from build123d import *

# Parameters (mm, degrees)
SKIZZE1_W                       = 35
SKIZZE1_H                       = 35
AUFSATZ_LINEAR_AUSTRAGEN1_DEPTH = 34
SKIZZE2_R                       = 16
AUFSATZ_LINEAR_AUSTRAGEN2_DEPTH = 35.8
SKIZZE3_R                       = 9.5
AUFSATZ_LINEAR_AUSTRAGEN3_DEPTH = 2
SKIZZE4_R                       = 3
AUFSATZ_LINEAR_AUSTRAGEN4_DEPTH = 18
SKIZZE5_R                       = 1.5
SCHNITT_LINEAR_AUSTRAGEN1_DEPTH = 4
FASE1_SIZE                      = 3
AUFSATZ_LINEAR_START            = 0.5
AUFSATZ_LINEAR_AUSTRAGEN5_DEPTH = 4.5
SCHNITT_LINEAR_AUSTRAGEN2_DEPTH = 12


with BuildPart() as part:
    # Skizze1 → Aufsatz-Linear austragen1 (new body)
    with BuildSketch(Plane.XY):
        Rectangle(SKIZZE1_W, SKIZZE1_H)
    extrude(amount=AUFSATZ_LINEAR_AUSTRAGEN1_DEPTH)

    # Skizze2 → Aufsatz-Linear austragen2 (add)
    with BuildSketch(Plane.XY.offset(34)):
        Circle(SKIZZE2_R)
    extrude(amount=AUFSATZ_LINEAR_AUSTRAGEN2_DEPTH)

    # Skizze3 → Aufsatz-Linear austragen3 (add)
    with BuildSketch(Plane.XY.offset(69.8)):
        Circle(SKIZZE3_R)
    extrude(amount=AUFSATZ_LINEAR_AUSTRAGEN3_DEPTH)

    # Skizze4 → Aufsatz-Linear austragen4 (add)
    with BuildSketch(Plane.XY.offset(69.8)):
        Circle(SKIZZE4_R)
    extrude(amount=AUFSATZ_LINEAR_AUSTRAGEN4_DEPTH)

    # Skizze5 → Schnitt-Linear austragen1 (cut)
    with BuildSketch(Plane.XY.offset(69.8)):
        with Locations((0, 13)):
            Circle(SKIZZE5_R)
        with Locations((13, 0)):
            Circle(SKIZZE5_R)
        with Locations((-13, 0)):
            Circle(SKIZZE5_R)
        with Locations((0, -13)):
            Circle(SKIZZE5_R)
    extrude(amount=-SCHNITT_LINEAR_AUSTRAGEN1_DEPTH, mode=Mode.SUBTRACT)

    # Fase1
    fase1_edges = [part.edges().sort_by_distance(p)[0] for p in [
        (-17.5, 17.5, 17),
        (17.5, 17.5, 17),
        (17.5, -17.5, 17),
        (-17.5, -17.5, 17),
    ]]
    chamfer(fase1_edges, length=FASE1_SIZE)

    # Skizze6 → Aufsatz-Linear austragen5 (add)
    with BuildSketch(Plane.XY.offset(34).offset(AUFSATZ_LINEAR_START)):
        Polygon((-17.5, 14.5), (-17.5, -14.5), (-14.5, -17.5), (14.5, -17.5), (17.5, -14.5), (17.5, 14.5), (14.5, 17.5), (-14.5, 17.5), align=None)
    extrude(amount=AUFSATZ_LINEAR_AUSTRAGEN5_DEPTH)

    # Skizze7 → Schnitt-Linear austragen2 (cut)
    with BuildSketch(Plane.XY.offset(87.8)):
        with BuildLine():
            Line((2, 2.236067977), (2, -2.236067977))
            ThreePointArc((2, -2.236067977), (3, 0), (2, 2.236067977))
        make_face()
    extrude(amount=-SCHNITT_LINEAR_AUSTRAGEN2_DEPTH, mode=Mode.SUBTRACT)


solid = part.part
Verification items for the finished model (mm, model axes). A direction names the side the tool comes from. Coordinates: 2 decimals unless noted, no trailing zeros. Loops run counter-clockwise (first coordinate to the right, second up) from the corner with the lowest first, then second, coordinate; pieces in that order, holes last. Notation, with made-up numbers: (9, -18.5) -> (23, -18.5) arc R28 ccw to (23, 6.5) -> close; hole circle Ø6 at (48.5, 88). An arc over 180 degrees is marked (long way). Answer as a JSON object with one key per item and string values. Group by question number.
Item 1: Sectioned sample at C-C on z = 59. Record the boundary of the cut face in (x, y).
Item 2: Scan lines: probe 1 along Y at (x, z) = (0, 68); probe 2 along Z at (x, y) = (-16, -3.5); probe 3 along Z at (x, y) = (-4, 14.5). Record each from-to range of solid material in increasing order.
Item 3: Sectioned sample at D-D on y = -8. Record the boundary of the cut face in (x, z), plus the area to 3 significant figures.
Item 4: Tool access check on faces 1 (the flat face through (-5.3, -15.5, 34.5)), 2 (the cylindrical face through (-0.325, 11.536, 67.828)), 3 (the flat face through (-16, 16, 37)). Record the directions out of +Z, -Z, +X, -X, +Y, -Y that give a thin tool (end or side, any length) a straight path to the whole face; none if there is none.
Item 5: Mould release check, pull along Z, two halves, no side actions. Record for faces 4 (the cylindrical face through (-3.47, -15.62, 34.25)), 5 (the flat face through (-13, 0, 65.8)), 6 (the cylindrical face through (-0.325, -14.464, 67.828)): +Z half, -Z half, draft (parallel to the pull), parting line (faces both ways), or undercut.
Item 6: Depth check by flat-ended pin: pin 1 (1.5 mm diameter, centred on x = -13, y = -6, fed in from +Z); pin 2 (1.5 mm diameter, centred on x = -5.5, z = 48, fed in from +Y); pin 3 (5 mm diameter, centred on x = -10, z = 46, fed in from -Y). Enter the tip coordinate at first touch or a pass-through.
Evaluation:
{
 "1": {"outline": "circle Ø32 at (0, 0)"},
 "2": {"probe 1": "y = -16 to -14.5, -11.5 to 11.5, 14.5 to 16", "probe 2": "z = 0 to 34, 34.5 to 39", "probe 3": "z = 0 to 69.8"},
 "3": {"outline": "(-17.5, 0) -> (17.5, 0) -> (17.5, 34) -> (13.86, 34) -> (13.86, 34.5) -> (17.5, 34.5) -> (17.5, 39) -> (13.86, 39) -> (13.86, 69.8) -> (5.12, 69.8) -> (5.12, 71.8) -> (-5.12, 71.8) -> (-5.12, 69.8) -> (-13.86, 69.8) -> (-13.86, 39) -> (-17.5, 39) -> (-17.5, 34.5) -> (-13.86, 34.5) -> (-13.86, 34) -> (-17.5, 34) -> close", "area": "2,240 mm²"},
 "4": {"face 1": "none", "face 2": "+Z", "face 3": "+Z, -Z, -X, +Y"},
 "5": {"face 4": "undercut", "face 5": "+Z half", "face 6": "draft"},
 "6": {"pin 1": "stops at z = 69.8", "pin 2": "stops at y = 15.28", "pin 3": "stops at y = -14.13"}
}
